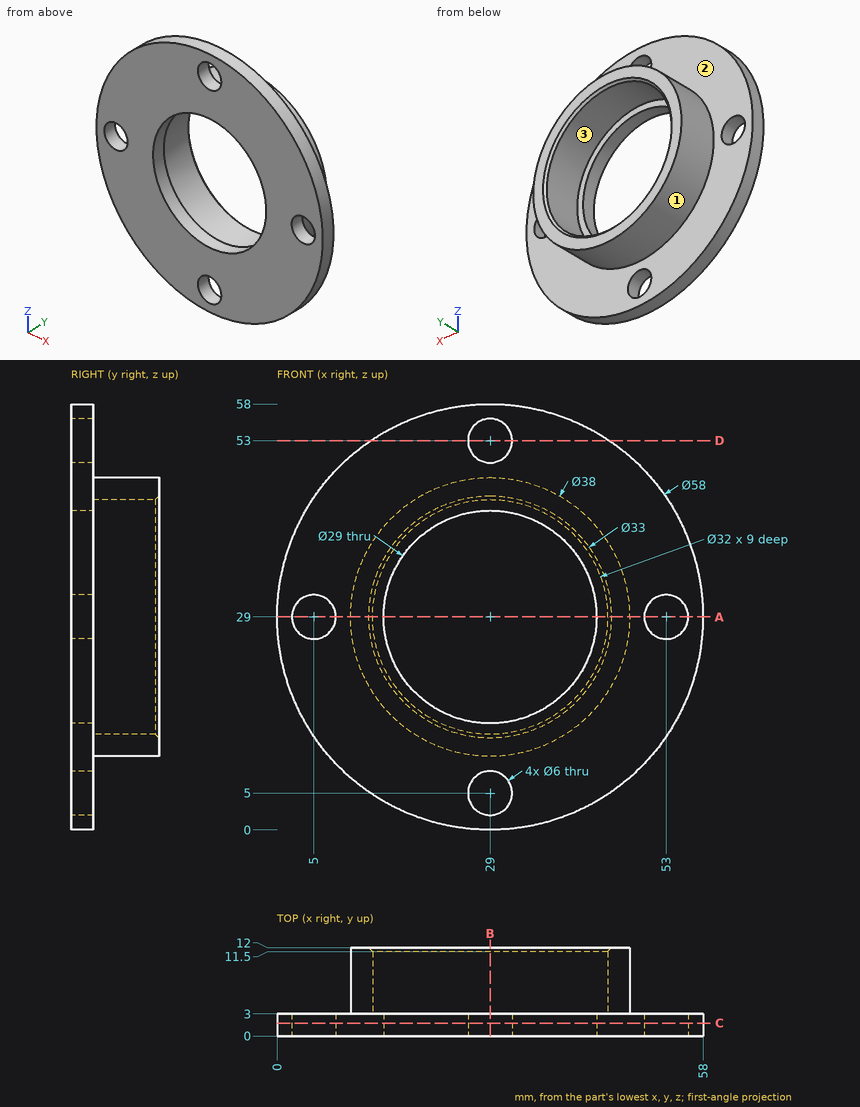
For this review, use the dimensioned drawing (mm, ordinates from the lowest corner) and the shaded views. Give positions to 0.01 mm unless a question says otherwise; leave off trailing zeros. Loops run counter-clockwise (first coordinate to the right, second up) from the corner with the lowest first, then second, coordinate; pieces in that order, holes last. Notation, with made-up numbers: (78.5, -22.75) -> (129.5, -22.75) arc R18 cw to (129.5, 10.25) -> close; hole circle Ø6 at (73, -37.5). An arc over 180 degrees is marked (long way). One line per question, with ' | ' between items. Start each with the question number.
(1) We need section D-D (z = 53). State the section outline as (x, y) points, and give its area (3 significant figures).
(2) We need section B-B (x = 29). State the section outline as (y, z) points, and give its area (3 significant figures).
(3) Draft analysis for pull direction Z (two halves, no side actions). For the marked faces 1, 2 and 3, state which applies: +Z half, -Z half, draft (parallel to the pull), parting line (faces both ways), or undercut.
(4) For line 1 (X direction, y = 1.35, z = 29); line 2 (X direction, y = 7, z = 29); line 3 (Y direction, x = 39, z = 52.5), list the stretches that pass through material, from the lowest coordinate up.
(5) Insertion check: P1, Ø1, axis at x = 9, y = 2, coming from the -Z side; P2, Ø9.5, axis at x = 29, z = 53, coming from the +Y side; P3, Ø1, axis at x = 45, y = 8, coming from the +Z side. Each pin has a flat end and moves straight along its axis. Give the tip position at first contact, or say it passes through.
(6) We need section C-C (y = 1.75). State the section outline as (x, z) points, and give its area (3 significant figures).
(7) We need section A-A (z = 29). State the section outline as (x, y) points.
The answers:
1) outline: (12.72, 0) -> (26, 0) -> (26, 3) -> (12.72, 3) -> close; (32, 0) -> (45.28, 0) -> (45.28, 3) -> (32, 3) -> close | area: 79.7 mm^2
2) outline: (0, 0) -> (3, 0) -> (3, 2) -> (0, 2) -> close; (0, 8) -> (3, 8) -> (3, 10) -> (12, 10) -> (12, 12.5) -> (11.5, 13) -> (3, 13) -> (3, 14.5) -> (0, 14.5) -> close; (0, 43.5) -> (3, 43.5) -> (3, 45) -> (11.5, 45) -> (12, 45.5) -> (12, 48) -> (3, 48) -> (3, 50) -> (0, 50) -> close; (0, 56) -> (3, 56) -> (3, 58) -> (0, 58) -> close | area: 105 mm^2
3) face 1: parting line | face 2: draft | face 3: undercut
4) line 1: x = 0 to 2, 8 to 14.5, 43.5 to 50, 56 to 58 | line 2: x = 10 to 13, 45 to 48 | line 3: y = 0 to 3
5) P1: stops at z = 7.53 | P2: stops at y = 3 | P3: stops at z = 39.99
6) outline: circle Ø58 at (29, 29); hole circle Ø6 at (5, 29); hole circle Ø29 at (29, 29); hole circle Ø6 at (29, 5); hole circle Ø6 at (29, 53); hole circle Ø6 at (53, 29) | area: 1,870 mm^2
7) outline: (0, 0) -> (2, 0) -> (2, 3) -> (0, 3) -> close; (8, 0) -> (14.5, 0) -> (14.5, 3) -> (13, 3) -> (13, 11.5) -> (12.5, 12) -> (10, 12) -> (10, 3) -> (8, 3) -> close; (43.5, 0) -> (50, 0) -> (50, 3) -> (48, 3) -> (48, 12) -> (45.5, 12) -> (45, 11.5) -> (45, 3) -> (43.5, 3) -> close; (56, 0) -> (58, 0) -> (58, 3) -> (56, 3) -> close
